from build123d import *

# Parameters (mm, degrees)
SKETCH1_R                    = 95
BOSS_EXTRUDE1_DEPTH          = 6.35
BOSS_EXTRUDE2_START          = -6.35
BOSS_EXTRUDE2_DEPTH          = 6.35
SKETCH4_R                    = 72.75
CUT_EXTRUDE2_DEPTH           = 3
CUT_EXTRUDE3_REACH           = 152.749
SKETCH5_R                    = 17.5
TAP_DRILL_FOR_M10X1_5_TAP1_D = 8.5
CUT_EXTRUDE4_REACH           = 152.845
SKETCH3_R                    = 2.6162
BOSS_EXTRUDE3_START          = -6.35
BOSS_EXTRUDE3_DEPTH          = 6.35
CUT_EXTRUDE5_REACH           = 181.824
SKETCH9_R                    = 2.6162
FILLET1_R                    = 20
FILLET2_R                    = 5


with BuildPart() as part:
    # Sketch1 → Boss-Extrude1 (new body)
    with BuildSketch(Plane.XY):
        Circle(SKETCH1_R)
    extrude(amount=BOSS_EXTRUDE1_DEPTH)

    # Sketch2 → Boss-Extrude2 (add)
    with BuildSketch(Plane.XY.offset(6.35).offset(BOSS_EXTRUDE2_START)):
        with BuildLine():
            Line((87.946, -117), (-87.946, -117))
            Line((-87.946, -117), (-87.946, -35.923544981))
            ThreePointArc((-87.946, -35.923544981), (0, -95), (87.946, -35.923544981))
            Line((87.946, -35.923544981), (87.946, -117))
        make_face()
    extrude(amount=BOSS_EXTRUDE2_DEPTH)

    # Sketch4 → Cut-Extrude2 (cut)
    with BuildSketch(Plane.XY.offset(6.35)):
        Circle(SKETCH4_R)
    extrude(amount=-CUT_EXTRUDE2_DEPTH, mode=Mode.SUBTRACT)

    # Sketch5 → Cut-Extrude3 (cut, up to next)
    with BuildSketch(Plane.XY.offset(3.35), mode=Mode.PRIVATE) as cut_extrude3_sk1:
        Circle(SKETCH5_R)
    cut_extrude3_tool1 = extrude(cut_extrude3_sk1.sketch, amount=-CUT_EXTRUDE3_REACH, mode=Mode.PRIVATE) & part.part
    add(cut_extrude3_tool1.solids().sort_by_distance((0, 0, 3.35))[0], mode=Mode.SUBTRACT)

    # Tap Drill for M10x1.5 Tap1 (through all)
    with Locations(Plane(origin=(0, 85, 6.35), x_dir=(1, 0, 0), z_dir=(0, 0, 1))):
        with Locations((0, 0), (73.612159322, -42.5), (73.612159322, -127.5), (0, -170), (-73.612159322, -127.5), (-73.612159322, -42.5)):
            Hole(TAP_DRILL_FOR_M10X1_5_TAP1_D / 2)

    # Sketch3 → Cut-Extrude4 (cut, up to next)
    with BuildSketch(Plane.XY.offset(6.35), mode=Mode.PRIVATE) as cut_extrude4_sk1:
        with Locations((-77.946, -107)):
            Circle(SKETCH3_R)
    cut_extrude4_tool1 = extrude(cut_extrude4_sk1.sketch, amount=-CUT_EXTRUDE4_REACH, mode=Mode.PRIVATE) & part.part
    # Sketch3 → Cut-Extrude4 (cut, up to next)
    with BuildSketch(Plane.XY.offset(6.35), mode=Mode.PRIVATE) as cut_extrude4_sk2:
        with Locations((77.946, -107)):
            Circle(SKETCH3_R)
    cut_extrude4_tool2 = extrude(cut_extrude4_sk2.sketch, amount=-CUT_EXTRUDE4_REACH, mode=Mode.PRIVATE) & part.part
    # Sketch3 → Cut-Extrude4 (cut, up to next)
    with BuildSketch(Plane.XY.offset(6.35), mode=Mode.PRIVATE) as cut_extrude4_sk3:
        with Locations((0, -107)):
            Circle(SKETCH3_R)
    cut_extrude4_tool3 = extrude(cut_extrude4_sk3.sketch, amount=-CUT_EXTRUDE4_REACH, mode=Mode.PRIVATE) & part.part
    add(cut_extrude4_tool1.solids().sort_by_distance((-77.946, -107, 6.35))[0], mode=Mode.SUBTRACT)
    add(cut_extrude4_tool2.solids().sort_by_distance((77.946, -107, 6.35))[0], mode=Mode.SUBTRACT)
    add(cut_extrude4_tool3.solids().sort_by_distance((0, -107, 6.35))[0], mode=Mode.SUBTRACT)

    # Sketch8 → Boss-Extrude3 (add)
    with BuildSketch(Plane.XY.offset(6.35).offset(BOSS_EXTRUDE3_START)):
        with BuildLine():
            Line((87.946, 152.5499), (-87.946, 152.5499))
            Line((-87.946, 152.5499), (-87.946, 35.923544981))
            ThreePointArc((-87.946, 35.923544981), (0, 95), (87.946, 35.923544981))
            Line((87.946, 35.923544981), (87.946, 152.5499))
        make_face()
    extrude(amount=BOSS_EXTRUDE3_DEPTH)

    # Sketch9 → Cut-Extrude5 (cut, up to next)
    with BuildSketch(Plane.XY.offset(6.35), mode=Mode.PRIVATE) as cut_extrude5_sk1:
        with Locations((-77.946, 142.5499)):
            Circle(SKETCH9_R)
    cut_extrude5_tool1 = extrude(cut_extrude5_sk1.sketch, amount=-CUT_EXTRUDE5_REACH, mode=Mode.PRIVATE) & part.part
    # Sketch9 → Cut-Extrude5 (cut, up to next)
    with BuildSketch(Plane.XY.offset(6.35), mode=Mode.PRIVATE) as cut_extrude5_sk2:
        with Locations((-77.946, 122.5499)):
            Circle(SKETCH9_R)
    cut_extrude5_tool2 = extrude(cut_extrude5_sk2.sketch, amount=-CUT_EXTRUDE5_REACH, mode=Mode.PRIVATE) & part.part
    # Sketch9 → Cut-Extrude5 (cut, up to next)
    with BuildSketch(Plane.XY.offset(6.35), mode=Mode.PRIVATE) as cut_extrude5_sk3:
        with Locations((77.946, 122.5499)):
            Circle(SKETCH9_R)
    cut_extrude5_tool3 = extrude(cut_extrude5_sk3.sketch, amount=-CUT_EXTRUDE5_REACH, mode=Mode.PRIVATE) & part.part
    # Sketch9 → Cut-Extrude5 (cut, up to next)
    with BuildSketch(Plane.XY.offset(6.35), mode=Mode.PRIVATE) as cut_extrude5_sk4:
        with Locations((77.946, 142.5499)):
            Circle(SKETCH9_R)
    cut_extrude5_tool4 = extrude(cut_extrude5_sk4.sketch, amount=-CUT_EXTRUDE5_REACH, mode=Mode.PRIVATE) & part.part
    add(cut_extrude5_tool1.solids().sort_by_distance((-77.946, 142.5499, 6.35))[0], mode=Mode.SUBTRACT)
    add(cut_extrude5_tool2.solids().sort_by_distance((-77.946, 122.5499, 6.35))[0], mode=Mode.SUBTRACT)
    add(cut_extrude5_tool3.solids().sort_by_distance((77.946, 122.5499, 6.35))[0], mode=Mode.SUBTRACT)
    add(cut_extrude5_tool4.solids().sort_by_distance((77.946, 142.5499, 6.35))[0], mode=Mode.SUBTRACT)

    # Fillet1
    fillet1_edges = [part.edges().sort_by_distance(p)[0] for p in [
        (-87.946, -35.923544981, 3.175),
        (87.946, -35.923544981, 3.175),
        (-87.946, 35.923544981, 3.175),
        (87.946, 35.923544981, 3.175),
    ]]
    fillet(fillet1_edges, radius=FILLET1_R)

    # Fillet2
    fillet2_edges = [part.edges().sort_by_distance(p)[0] for p in [
        (-87.946, -117, 3.175),
        (87.946, -117, 3.175),
        (-87.946, 152.5499, 3.175),
        (87.946, 152.5499, 3.175),
    ]]
    fillet(fillet2_edges, radius=FILLET2_R)


solid = part.part
Work out the finished part from the listing and answer in its coordinate system (mm). A direction names the side the tool comes from. Give positions to 0.01 mm unless a question says otherwise; leave off trailing zeros. Loops run counter-clockwise (first coordinate to the right, second up) from the corner with the lowest first, then second, coordinate; pieces in that order, holes last. Notation, with made-up numbers: (11.5, 83) -> (39.5, 83) arc R30 cw to (39.5, 108) -> close; hole circle Ø4 at (69.25, 70). An arc over 180 degrees is marked (long way). Use a Markdown table: item, result. Add a question column.
1. Section D-D on z = 1.25 is taken. State how many separate pieces and enclosed holes the cut face has, and give its area (3 significant figures).
2. Section A-A on y = 0 is taken. Determine the outline of the cut face in (x, z).
3. Find the intervals of material crossed by probe 1 along Y at (x, z) = (0, 4.75); probe 2 along Y at (x, z) = (0, 2.5); probe 3 along Z at (x, y) = (-34.5, 12), in increasing order.
4. Section B-B on x = 9 is taken. Determine the outline of the cut face in (y, z), and give its area (3 significant figures).
5. Section C-C on y = 85 is taken. Determine the outline of the cut face in (x, z), and give its area (3 significant figures).
6. Determine the mould class of faces 1 (the cylindrical face through (-77.666, -41.223, 3.131)), 2 (the cylindrical face through (-86.52, 151.046, 3.219)), 3 (the flat face through (1, -117, 3)) for opening direction X: released by +X, released by -X, zero draft, split by the parting line, or undercut.
7. Flat-ended cylindrical pins translate along their axes: pin 1 Ø3 at (y, z) = (-77, 4.5) entering from -X; pin 2 Ø3 at (x, y) = (-77.95, 142.55) entering from +Z; pin 3 Ø6 at (x, y) = (-77.946, -107) entering from +Z; pin 4 Ø1.5 at (y, z) = (52, 3) entering from +X. Find the tip coordinate at first contact, or state that the pin passes through.
8. For faces 4 (the cylindrical face through (-88.264, 36.106, 3.219)), 5 (the flat face through (87.946, 93, 3)), 6 (the flat face through (87.946, -75, 3)), determine the directions among +Z, -Z, +X, -X, +Y, -Y from which every point of the face is accessible in a straight line to the end or side of a thin tool.
Results below:
| question | item | result |
|---|---|---|
| 1 | separate pieces | 1 |
| 1 | enclosed holes | 14 |
| 1 | area | 46,600 mm^2 |
| 2 | outline | (-95, 0) -> (-17.5, 0) -> (-17.5, 3.35) -> (-72.75, 3.35) -> (-72.75, 6.35) -> (-95, 6.35) -> close; (17.5, 0) -> (95, 0) -> (95, 6.35) -> (72.75, 6.35) -> (72.75, 3.35) -> (17.5, 3.35) -> close |
| 3 | probe 1 | y = -117 to -109.62, -104.38 to -89.25, -80.75 to -72.75, 72.75 to 80.75, 89.25 to 152.55 |
| 3 | probe 2 | y = -117 to -109.62, -104.38 to -89.25, -80.75 to -17.5, 17.5 to 80.75, 89.25 to 152.55 |
| 3 | probe 3 | z = 0 to 3.35 |
| 4 | outline | (-117, 0) -> (-15.01, 0) -> (-15.01, 3.35) -> (-72.19, 3.35) -> (-72.19, 6.35) -> (-117, 6.35) -> close; (15.01, 0) -> (152.55, 0) -> (152.55, 6.35) -> (72.19, 6.35) -> (72.19, 3.35) -> (15.01, 3.35) -> close |
| 4 | area | 1,180 mm^2 |
| 5 | outline | (-87.95, 0) -> (-4.25, 0) -> (-4.25, 6.35) -> (-87.95, 6.35) -> close; (4.25, 0) -> (87.95, 0) -> (87.95, 6.35) -> (4.25, 6.35) -> close |
| 5 | area | 1,060 mm^2 |
| 6 | face 1 | undercut |
| 6 | face 2 | released by -X |
| 6 | face 3 | zero draft |
| 7 | pin 1 | stops at x = -87.95 |
| 7 | pin 2 | passes through |
| 7 | pin 3 | stops at z = 6.35 |
| 7 | pin 4 | stops at x = 87.95 |
| 8 | face 4 | +Z, -Z, -X, +Y |
| 8 | face 5 | +Z, -Z, +X, +Y |
| 8 | face 6 | +Z, -Z, +X, -Y |
